Verification items for the finished model (mm, model axes). Give positions to 0.01 mm unless a question says otherwise; leave off trailing zeros. Write each loop counter-clockwise with the first axis right and the second up, starting at its lowest first coordinate (ties: lowest second). Pieces come first, ordered by that corner, then holes.
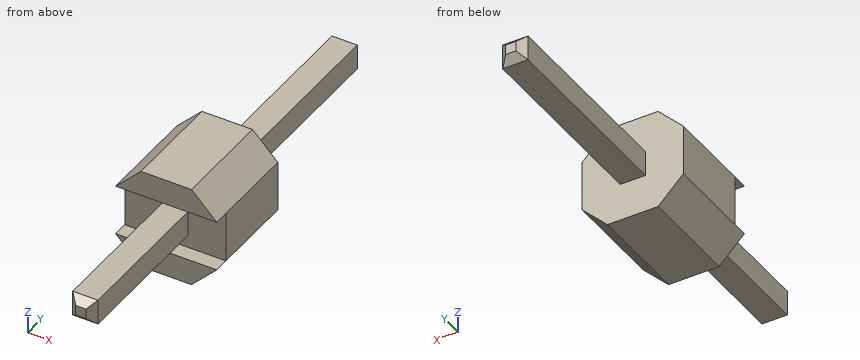
from build123d import *

# Parameters (mm, degrees)
BOSS_EXTRUDE1_DEPTH = 2.54
SKETCH2_W           = 1.27
SKETCH2_H           = 0.381
CUT_EXTRUDE1_DEPTH  = 2.54
SKETCH3_W           = 0.635
SKETCH3_H           = 0.635
BOSS_EXTRUDE2_DEPTH = 5.08
CHAMFER1_SIZE       = 0.1905
SKETCH4_W           = 0.635
SKETCH4_H           = 0.635
BOSS_EXTRUDE3_DEPTH = 3.937
CHAMFER2_SIZE       = 0.1905


with BuildPart() as part:
    # Sketch1 → Boss-Extrude1 (new body)
    with BuildSketch(Plane(origin=(0, 0, 0), x_dir=(1, 0, 0), z_dir=(0, 1, 0))):
        Polygon((0.635, 1.27), (1.27, 0.635), (1.27, -0.635), (0.635, -1.27), (-0.635, -1.27), (-1.27, -0.635), (-1.27, 0.635), (-0.635, 1.27), align=None)
    extrude(amount=BOSS_EXTRUDE1_DEPTH)

    # Sketch2 → Cut-Extrude1 (cut)
    with BuildSketch(Plane(origin=(1.27, 0, 0), x_dir=(0, 0, -1), z_dir=(1, 0, 0))):
        with Locations((0, 0.1905)):
            Rectangle(SKETCH2_W, SKETCH2_H)
    extrude(amount=-CUT_EXTRUDE1_DEPTH, mode=Mode.SUBTRACT)

    # Sketch3 → Boss-Extrude2 (add)
    with BuildSketch(Plane(origin=(0, 2.54, 0), x_dir=(1, 0, 0), z_dir=(0, 1, 0))):
        Rectangle(SKETCH3_W, SKETCH3_H)
    extrude(amount=BOSS_EXTRUDE2_DEPTH)

    # Chamfer1
    chamfer1_edges = [part.edges().sort_by_distance(p)[0] for p in [
        (0.3175, 7.62, 0),
        (0, 7.62, -0.3175),
        (-0.3175, 7.62, 0),
        (0, 7.62, 0.3175),
    ]]
    chamfer(chamfer1_edges, length=CHAMFER1_SIZE)

    # Sketch4 → Boss-Extrude3 (add)
    with BuildSketch(Plane.XZ.offset(-0.381)):
        Rectangle(SKETCH4_W, SKETCH4_H)
    extrude(amount=BOSS_EXTRUDE3_DEPTH)

    # Chamfer2
    chamfer2_edges = [part.edges().sort_by_distance(p)[0] for p in [
        (0.3175, -3.556, 0),
        (0, -3.556, 0.3175),
        (-0.3175, -3.556, 0),
        (0, -3.556, -0.3175),
    ]]
    chamfer(chamfer2_edges, length=CHAMFER2_SIZE)


solid = part.part
Item 1: Sectioned sample at A-A on y = 0.25. Record the cut outline in (x, z) (1 decimal).
Answer key:
outline: (-1.3, -0.6) - (-0.6, -1.3) - (0.6, -1.3) - (1.3, -0.6) - close; (-1.3, 0.6) - (1.3, 0.6) - (0.6, 1.3) - (-0.6, 1.3) - close; (-0.3, -0.3) - (0.3, -0.3) - (0.3, 0.3) - (-0.3, 0.3) - close
Item 2: Scan lines: line 1 along Y through (x, z) = (-1.1, 0.35); line 2 along Y through (x, z) = (-0.9, 0.7); line 3 along X through (y, z) = (3, -0.25). Record each from-to range of solid material in increasing order.
Answer key:
line 1: y = 0.38 to 2.54
line 2: y = 0 to 2.54
line 3: x = -0.32 to 0.32
Item 3: Depth check by flat-ended pin: pin 1 (0.7 mm diameter, centred on y = 6, z = 0, fed in from +X); pin 2 (0.5 mm diameter, centred on x = 0, y = 5, fed in from -Z); pin 3 (0.7 mm diameter, centred on y = -1.5, z = 0, fed in from -X). Enter the tip coordinate at first touch or a pass-through.
Answer key:
pin 1: stops at x = 0.32
pin 2: stops at z = -0.32
pin 3: stops at x = -0.32
Item 4: Sectioned sample at C-C on z = 0. Record the cut outline in (x, y).
Answer key:
outline: (-1.27, 0.38) - (-0.32, 0.38) - (-0.32, -3.37) - (-0.13, -3.56) - (0.13, -3.56) - (0.32, -3.37) - (0.32, 0.38) - (1.27, 0.38) - (1.27, 2.54) - (0.32, 2.54) - (0.32, 7.43) - (0.13, 7.62) - (-0.13, 7.62) - (-0.32, 7.43) - (-0.32, 2.54) - (-1.27, 2.54) - close
Item 5: Sectioned sample at D-D on y = -2.5. Record the cut outline in (x, z).
Answer key:
outline: (-0.32, -0.32) - (0.32, -0.32) - (0.32, 0.32) - (-0.32, 0.32) - close
